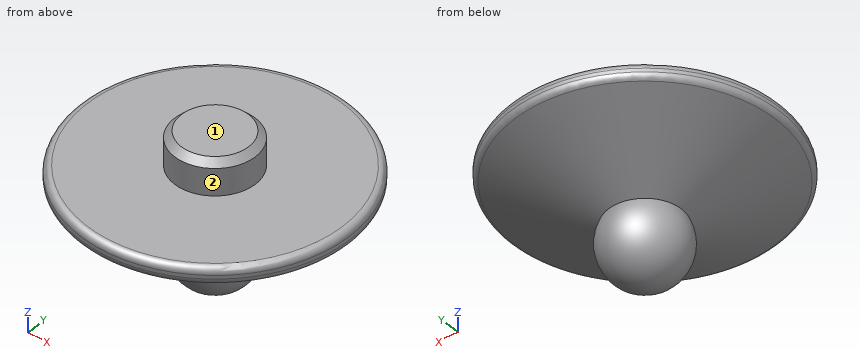
```python
from build123d import *

# Parameters (mm, degrees)
SKETCH_1_R      = 6
EXTRUDE_1_DEPTH = 5
CHAMFER_1_SIZE  = 1
FILLET_1_R      = 1


with BuildPart() as part:
    # 草图1 → 凸台-拉伸1 (new body)
    with BuildSketch(Plane.XY):
        Circle(SKETCH_1_R)
    extrude(amount=EXTRUDE_1_DEPTH)

    # 草图2 → 旋转1 (revolve)
    with BuildSketch(Plane(origin=(0, 0, 0), x_dir=(0, 0, -1), z_dir=(1, 0, 0)), mode=Mode.PRIVATE) as revolve_1_sk:
        with BuildLine():
            Line((0, 0), (0, 20))
            Line((0, 20), (2.174, 20))
            Line((2.174, 20), (8.964324636, 5.437862673))
            ThreePointArc((8.964324636, 5.437862673), (14.723813566, 5.060338535), (17.5, 0))
            Line((17.5, 0), (0, 0))
        make_face()
    revolve(revolve_1_sk.sketch.rotate(Axis((0, 0, 0), (0, 0, -1)), 90), axis=Axis((0, 0, 0), (0, 0, -1)))

    # 倒角1
    chamfer_1_edges = [part.edges().sort_by_distance(p)[0] for p in [
        (-6, 0, 5),
    ]]
    chamfer(chamfer_1_edges, length=CHAMFER_1_SIZE)

    # 圆角1
    fillet_1_edges = [part.edges().sort_by_distance(p)[0] for p in [
        (-20, 0, -2.174),
        (-20, 0, 0),
    ]]
    fillet(fillet_1_edges, radius=FILLET_1_R)


solid = part.part
```
Input: part model. Units: mm. Frame: model coordinates. Face numbers are marked on the shaded views. A direction names the side the tool comes from. Give positions to 0.01 mm unless a question says otherwise; leave off trailing zeros. Order: outer loops, then holes, each group sorted by start corner. A loop starts at its lowest first (then second) coordinate and runs counter-clockwise, first axis right, second up.
1. Cut plane A-A (z = 0.5). Return loops of the section in (x, y), and give its area (3 significant figures).
Computed:
outline: circle Ø12 at (0, 0)
area: 113 mm2
2. Line query: probe 1 along Z at (x, y) = (-1, 7); probe 2 along Z at (x, y) = (-9, -13); probe 3 along Y at (x, z) = (-1, -8.25). Output: solid intervals per line, ascending.
Computed:
probe 1: z = -8.2 to 0
probe 2: z = -4.13 to 0
probe 3: y = -6.9 to 6.9
3. Cut plane B-B (z = -4.75). Return loops of the section in (x, y).
Computed:
outline: circle Ø28.95 at (0, 0)
4. Pin query (flat end, axial travel): pin 1 Ø6 at (x, y) = (10, -7.5) entering from +Z; pin 2 Ø12 at (x, y) = (-8.5, -5) entering from -Z; pin 3 Ø1.5 at (y, z) = (10.5, -3) entering from +X. Return the tip coordinate at first contact, or that it passes through.
Computed:
pin 1: stops at z = 0
pin 2: stops at z = -16.09
pin 3: stops at x = 16.77
5. Set-up query: the marked faces 1 and 2. Return all of +Z, -Z, +X, -X, +Y, -Y with unobstructed straight access to the full face (end or side cutting, diameter ignored); none if empty.
Computed:
face 1: +Z, +X, -X, +Y, -Y
face 2: +Z
